For this review, take the finished solid that the model builds, in its own axes (mm). A direction names the side the tool comes from. Give positions to 0.01 mm unless a question says otherwise; leave off trailing zeros. Loops run counter-clockwise (first coordinate to the right, second up) from the corner with the lowest first, then second, coordinate; pieces in that order, holes last. Notation, with made-up numbers: M 28.25,38 L 52.25,38 A24 ccw 52.25,69 Z; hole C 52,75.25 d4. An arc over 180 degrees is marked long. Use CSV: the item, a comma, the result in double quotes. Start each with the question number.
1. Tool access review of faces 1 (the face through (27, -8, -70)), 2 (the face through (25.92, -6.48, 80.12)), 3 (the face through (-35, -8, -70)): name each direction out of +Z, -Z, +X, -X, +Y, -Y from which nothing blocks a thin tool from reaching the whole face with its end or side.
2. Take a section at A-A, the plane y = -19. Write out the cut boundary in (x, z).
3. The part is to be moulded in two halves that separate along X. For faces 4 (the face through (40, -17, -1)), 5 (the face through (23, -6, -67)), 6 (the face through (-40, -3, -38)), 7 (the face through (27, -8, 85)), say which applies: pulls with the +X half, pulls with the -X half, needs draft (parallel to the pull), parting line crosses it, or undercut.
4. Take a section at C-C, the plane z = 68.5. Write out the cut boundary in (x, y), and give its area (3 significant figures).
5. Take a section at B-B, the plane x = 24. Write out the cut boundary in (y, z).
6. To check wall thickness, follow line 1 (X direction, y = -9.5, z = -77.5); line 2 (X direction, y = -11.5, z = -73); line 3 (Y direction, x = 0, z = -64.5). State the ranges of each line that lie inside material, in increasing order. Write a range as [from, to].
7. Insertion check: P1, Ø5, axis at x = -37, z = -71, coming from the -Y side; P2, Ø1.5, axis at x = 8.5, y = -7.5, coming from the -Z side; P3, Ø1.5, axis at x = -37.5, y = -13, coming from the +Z side; P4, Ø5, axis at x = 18, z = 48, coming from the -Y side. Each pin has a flat end and moves straight along its axis. Give the tip position at first contact, or say it passes through.
8. Take a section at D-D, the plane x = 13.5. Write out the cut boundary in (y, z).
from build123d import *

# Parameters (mm, degrees)
SKETCH_W      = 80
SKETCH_H      = 200
PAD_DEPTH     = 5
SKETCH001_R   = 5
PAD001_DEPTH  = 3
SKETCH002_W   = 5
SKETCH002_H   = 200
SKETCH002_H_2 = 23
PAD002_DEPTH  = 30


with BuildPart() as part:
    # Sketch → Pad (new body)
    with BuildSketch(Plane.XZ):
        Rectangle(SKETCH_W, SKETCH_H)
    extrude(amount=PAD_DEPTH)

    # Sketch001 (on Face6 of Pad) → Pad001 (join)
    with BuildSketch(Plane.XZ.offset(5)):
        with Locations((-35, 85)):
            Circle(SKETCH001_R)
        with Locations((27, 85)):
            Circle(SKETCH001_R)
        with Locations((-35, -70)):
            Circle(SKETCH001_R)
        with Locations((27, -70)):
            Circle(SKETCH001_R)
    extrude(amount=PAD001_DEPTH)

    # Sketch002 (on Face5 of Pad001) → Pad002 (join)
    with BuildSketch(Plane.XZ.offset(5)):
        with Locations((37.5, 0)):
            Rectangle(SKETCH002_W, SKETCH002_H)
        with Locations((-37.5, -88.5)):
            Rectangle(SKETCH002_W, SKETCH002_H_2)
    extrude(amount=PAD002_DEPTH)


solid = part.part
Result set:
1,face 1,"+Z, -Z, -X, -Y"
1,face 2,"-Y"
1,face 3,"+Z, -X, -Y"
2,outline,"M -40,-100 L -35,-100 L -35,-77 L -40,-77 Z; M 35,-100 L 40,-100 L 40,100 L 35,100 Z"
3,face 4,"pulls with the +X half"
3,face 5,"undercut"
3,face 6,"pulls with the -X half"
3,face 7,"needs draft"
4,outline,"M -40,-5 L 35,-5 L 35,-35 L 40,-35 L 40,0 L -40,0 Z"
4,area,"550 mm2"
5,outline,"M -8,-74 L -5,-74 L -5,-100 L 0,-100 L 0,100 L -5,100 L -5,89 L -8,89 L -8,81 L -5,81 L -5,-66 L -8,-66 Z"
6,line 1,"[-40, -35], [35, 40]"
6,line 2,"[35, 40]"
6,line 3,"[-5, 0]"
7,P1,"y = -8"
7,P2,"through"
7,P3,"z = -77"
7,P4,"y = -5"
8,outline,"M -5,-100 L 0,-100 L 0,100 L -5,100 Z"
